Input: part model. Units: mm. Frame: model coordinates. A direction names the side the tool comes from. Round coordinates to 2 decimals unless told otherwise and drop trailing zeros. Order: outer loops, then holes, each group sorted by start corner. A loop starts at its lowest first (then second) coordinate and runs counter-clockwise, first axis right, second up. Notation, with made-up numbers: (6.25, 10.25) - (30.25, 10.25) arc R27 ccw to (30.25, 41.25) - close; hole circle Ø6 at (-28, 69.25). An arc over 180 degrees is marked (long way). One line per item, written item: value. Start each with the question number.
from build123d import *

# Parameters (mm, degrees)
F1_DEPTH = 30
F2_R     = 7.5
F3_DEPTH = 97.501
F4_R     = 10
F5_DEPTH = 5.001
F6_R     = 10


with BuildPart() as f1:
    # F0 (on Front) → F1 (new body)
    with BuildSketch(Plane.XZ):
        Polygon((0, 50), (0, 0), (-92.5, -410), (-92.5, -440), (-87.5, -440), (-87.5, -410), (5, 0), (5, 50), align=None)
    extrude(amount=F1_DEPTH)

    # F2 (on face) → F3 (cut, through all)
    with BuildSketch(Plane.YZ.offset(5)):
        with Locations((-15, 25)):
            Circle(F2_R)
    extrude(amount=-F3_DEPTH, mode=Mode.SUBTRACT)

    # F4 (on face) → F5 (cut, through all)
    with BuildSketch(Plane.YZ.offset(-87.5)):
        with Locations((-15, -425)):
            Circle(F4_R)
    extrude(amount=-F5_DEPTH, mode=Mode.SUBTRACT)

    # F6
    f6_edges = [f1.edges().sort_by_distance(p)[0] for p in [
        (-90, -30, -440),
        (-90, 0, -440),
        (2.5, -30, 50),
        (2.5, 0, 50),
    ]]
    fillet(f6_edges, radius=F6_R)


solid = f1.part
Item 1: Pull-direction query (Z, two-part tool) for faces 1 (the face through (-87.5, -18, -415)), 2 (the face through (-41.897, -14.79, -207.87)), 3 (the face through (-89.965, -16.302, -415.085)); classes: released by +Z, released by -Z, zero draft, split by the parting line, or undercut.
Item 2: Line query: L1, parallel to X at y = -22.5, z = 27; L2, parallel to X at y = -7.5, z = -44.5. Output: solid intervals per line, ascending.
Item 3: Section query D-D on x = -43. Return loops of the section in (y, z), and give its area (3 significant figures).
Item 4: Section query A-A on z = 25. Return loops of the section in (x, y).
Item 5: First-contact query: pin 1 Ø10 at (y, z) = (-19, -374.5) entering from +X; pin 2 Ø10 at (y, z) = (-6, -263) entering from -X; pin 3 Ø5 at (y, z) = (-15, -53.5) entering from +X. Flat tips, straight axial feed; report the tip coordinate or a pass-through.
Item 6: Section query C-C on z = -425. Return loops of the section in (x, y), and give its area (3 significant figures).
Item 7: Reachability of faces 4 (the face through (0, -21, 20)), 5 (the face through (2.46, -26.99, 47.15)) from +Z, -Z, +X, -X, +Y, -Y: full face, straight path, thin tool, end or side. Return the list, or none.
Item 8: Section query B-B on y = -15. Return loops of the section in (x, z), and give its area (4 significant figures).
Geometry results:
1. face 1: zero draft
1. face 2: released by -Z
1. face 3: undercut
2. L1: x = 0 to 5
2. L2: x = -10.04 to -5.04
3. outline: (-30, -212.76) - (0, -212.76) - (0, -190.59) - (-30, -190.59) - close
3. area: 665 mm^2
4. outline: (0, -30) - (5, -30) - (5, -22.5) - (0, -22.5) - close; (0, -7.5) - (5, -7.5) - (5, 0) - (0, 0) - close
5. pin 1: stops at x = -78.36
5. pin 2: stops at x = -60.46
5. pin 3: stops at x = -6.51
6. outline: (-92.5, -30) - (-87.5, -30) - (-87.5, -25) - (-92.5, -25) - close; (-92.5, -5) - (-87.5, -5) - (-87.5, 0) - (-92.5, 0) - close
6. area: 50.0 mm^2
7. face 4: +Z, -X, +Y, -Y
7. face 5: +Z, +X, -X, -Y
8. outline: (-92.5, -440) - (-87.5, -440) - (-87.5, -435) - (-92.5, -435) - close; (-92.5, -415) - (-87.5, -415) - (-87.5, -410) - (5, 0) - (5, 17.5) - (0, 17.5) - (0, 0) - (-92.5, -410) - close; (0, 32.5) - (5, 32.5) - (5, 50) - (0, 50) - close
8. area: 2,275 mm^2
